Work out the finished part from the listing and answer in its coordinate system (mm). Face numbers are marked on the shaded views. A direction names the side the tool comes from. Coordinates: 2 decimals unless noted, no trailing zeros. Order: outer loops, then holes, each group sorted by start corner. A loop starts at its lowest first (then second) coordinate and runs counter-clockwise, first axis right, second up. Notation, with made-up numbers: M 53.5,9.5 L 94.5,9.5 A22 cw 94.5,20.5 Z; hole C 55,52.5 d8. An arc over 180 degrees is marked long. Write item = value, one per line. Start each with the question number.
Q1. Find section C-C on y = 1.5. Give the vertices of the cut face in (x, z) (3 decimals).
Q2. Find section A-A on y = 7.5. Give the vertices of the cut face in (x, z) (3 decimals), and give its area (3 significant figures).
Q3. Find section D-D on y = 5.25. Give the vertices of the cut face in (x, z) (3 decimals).
Q4. A tool of negligible diameter and unlimited length cuts with its end or side. For the marked faces 1 and 2, from which of +Z, -Z, +X, -X, +Y, -Y can it reach the whole face along a straight path? Write none if from no direction.
Q5. Find section B-B on z = 4.25. Give the vertices of the cut face in (x, y), and give its area (3 significant figures).
Q6. Determine the mould class of the marked faces 3, 4 and 5 for opening direction X: released by +X, released by -X, zero draft, split by the parting line, or undercut.
Q7. Straight lines are drawn through the part: line 1 along Y through (x, z) = (0, 8.2); line 2 along Z through (x, y) = (-1.25, 3.25) (3 decimals); line 3 along Z through (x, y) = (-1.25, 2.25) (3 decimals). For each, find the intervals that lie inside material, in ascending order.
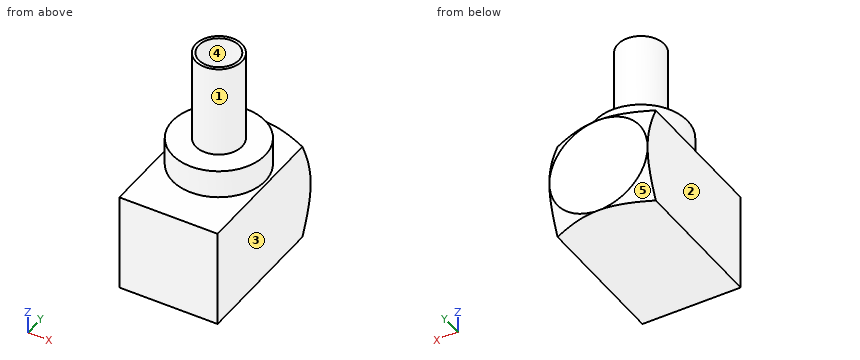
```python
from build123d import *

# Parameters (mm, degrees)
SKETCH_2_W      = 6.35
SKETCH_2_H      = 6.35
EXTRUDE_1_DEPTH = 10
SKETCH_6_R      = 3
EXTRUDE_2_DEPTH = 5
SKETCH_7_R      = 1.5
SKETCH_7_R_2    = 1.3
EXTRUDE_3_DEPTH = 6


with BuildPart() as part:
    # 草图2 → 凸台-拉伸1 (new body)
    with BuildSketch(Plane(origin=(0, 0, 0), x_dir=(1, 0, 0), z_dir=(0, 1, 0))):
        Rectangle(SKETCH_2_W, SKETCH_2_H)
    extrude(amount=EXTRUDE_1_DEPTH)

    # 草图5 → 切除-旋转1 (revolve, cut)
    with BuildSketch(Plane.XY):
        Polygon((3.175, 10), (5.248872861, 14.588450108), (5.248872861, 8.60417478), align=None)
    revolve(axis=Axis((0, 15.427678148, 0), (0, -1, 0)), mode=Mode.SUBTRACT)

    # 草图6 → 凸台-拉伸2 (add)
    with BuildSketch(Plane.XY):
        with Locations(Location((0, 5.416720089, 0), (0, 0, 180))):
            Circle(SKETCH_6_R)
    extrude(amount=EXTRUDE_2_DEPTH)

    # 草图7 → 凸台-拉伸3 (add)
    with BuildSketch(Plane.XY.offset(5)):
        with Locations((0, 5.416720089)):
            Circle(SKETCH_7_R)
        with Locations((0, 5.416720089)):
            Circle(SKETCH_7_R_2, mode=Mode.SUBTRACT)
    extrude(amount=EXTRUDE_3_DEPTH)


solid = part.part
```
Findings below:
q1.outline = M -3.175,-3.175 L 3.175,-3.175 L 3.175,3.175 L -3.175,3.175 Z
q2.outline = M -3.175,-3.175 L 3.175,-3.175 L 3.175,3.175 L 2.159,3.175 L 2.159,5 L -2.159,5 L -2.159,3.175 L -3.175,3.175 Z
q2.area = 48.2 mm^2
q3.outline = M -3.175,-3.175 L 3.175,-3.175 L 3.175,3.175 L 2.995,3.175 L 2.995,5 L 1.491,5 L 1.491,11 L 1.289,11 L 1.289,5 L -1.289,5 L -1.289,11 L -1.491,11 L -1.491,5 L -2.995,5 L -2.995,3.175 L -3.175,3.175 Z
q4.face_1 = +Z
q4.face_2 = +Z, -Z, -X, +Y, -Y
q5.outline = C 0,5.42 d6
q5.area = 28.3 mm^2
q6.face_3 = released by +X
q6.face_4 = undercut
q6.face_5 = released by -X
q7.line_1 = 3.92 to 4.12, 6.72 to 6.92
q7.line_2 = -3.175 to 5
q7.line_3 = -3.175 to 3.175
